Autodesk Inventor part; units mm, degrees
ref_plane "YZ Plane" through (0, 0, 0) normal (1, 0, 0) x (0, 1, 0)
ref_plane "XZ Plane" through (0, 0, 0) normal (0, 1, 0) x (-1, 0, 0)
ref_plane "XY Plane" through (0, 0, 0) normal (0, 0, 1) x (1, 0, 0)
sketch "Sketch1" plane through (0, 0, 0) normal (0, 1, 0) x (-1, 0, 0)
  line L0 (-13, -110) -> (13, -110)
  line L1 (13, -110) -> (13, 110)
  line L2 (13, 110) -> (-13, 110)
  line L3 (-13, 110) -> (-13, -110)
  line L4 (-13, -110) -> (13, 110) construction
  line L5 (13, -110) -> (-13, 110) construction
  point P0 (0, 0)
  dimension "d0" = 220
  dimension "d1" = 26
extrude "Extrusion1" add sketch "Sketch1" along normal blind 10
sketch "Sketch3" plane through (0, 0, 0) normal (0, -1, 0) x (1, 0, 0)
  line L0 (13, 110) -> (13, -110)
  line L1 (-13, -14) -> (13, -14)
  line L2 (13, -14) -> (13, 14)
  line L3 (13, 14) -> (-13, 14)
  line L4 (-13, 14) -> (-13, -14)
  line L5 (-13, -14) -> (13, 14) construction
  line L6 (13, -14) -> (-13, 14) construction
  point P0 (0, 0)
  dimension "d4" = 28
extrude "Extrusion2" add sketch "Sketch3" along normal blind 10
sketch "Sketch4" plane through (0, -10, 0) normal (0, -1, 0) x (1, 0, 0)
  line L0 (-10.125, 10.125) -> (10.125, 10.125)
  line L1 (10.125, 10.125) -> (10.125, -10.125)
  line L2 (10.125, -10.125) -> (-10.125, -10.125)
  line L3 (-10.125, -10.125) -> (-10.125, 10.125)
  line L4 (-10.125, 10.125) -> (10.125, -10.125) construction
  line L5 (10.125, 10.125) -> (-10.125, -10.125) construction
  point P0 (0, 0)
  dimension "d7" = 20.25
  dimension "d8" = 20.25
extrude "Extrusion3" cut sketch "Sketch4" against normal through all
sketch "Sketch5" plane through (-13, 0, 110) normal (-1, 0, 0) x (0, 0, 1)
  point P0 (-110, 0)
hole "Hole1" at (-13, 0, 0) direction (1, 0, 0) diameter 4.3 end through all
sketch "Sketch6" plane through (-13, 0, 110) normal (-1, 0, 0) x (0, 0, 1)
  circle A0 centre (-35, 0) radius 6.6
  line L0 (-96, 0) -> (0, 0)
  point P0 (-110, 0)
  dimension "d18" = 75
  dimension "d19" = 13.2
extrude "Extrusion4" cut sketch "Sketch6" against normal through all
sketch "Sketch7" plane through (0, 0, 0) normal (0, -1, 0) x (1, 0, 0)
  line L0 (-13, 81.6) -> (13, 81.6)
  line L1 (-13, 68.4) -> (-13, 81.6)
  line L2 (13, 68.4) -> (-13, 68.4)
  line L3 (13, 81.6) -> (13, 68.4)
  line L4 (0, 85) -> (0, 65)
  point P0 (0, 0)
  point P1 (0, 75)
  point P2 (13, 75)
  point P3 (0, 68.4)
  dimension "d22" = 20
hole "Hole2" at (0, 0, 65) at (0, 0, 85) direction (0, 1, 0) diameter 2.459 end through all
pattern_linear "Rectangular Pattern1" count 2 spacing 20 along (0, 0, 1) count 2 spacing 20 along (0, 0, -1) of "Extrusion4"
pattern_linear "Rectangular Pattern2" count 2 spacing 20 along (0, 0, 1) count 2 spacing 20 along (0, 0, -1) of "Hole2"
mirror "Mirror1" about plane through (0, 0, 0) normal (0, 0, 1) of "Extrusion4", "Hole2", "Rectangular Pattern1", "Rectangular Pattern2"
fillet "Fillet1" radius 5 2 edges at (0, 0, 14) (0, 0, -14)
properties part number "holder"
Geometry check sheet. Reference: the model listing, model coordinates, mm. A direction names the side the tool comes from. Coordinates: 2 decimals unless noted, no trailing zeros. Order: outer loops, then holes, each group sorted by start corner. A loop starts at its lowest first (then second) coordinate and runs counter-clockwise, first axis right, second up. Notation, with made-up numbers: (-4.75, 80) - (32.25, 80) arc R28 ccw to (32.25, 99) - close; hole circle Ø4 at (41, -35.75). An arc over 180 degrees is marked (long way). Answer in a Markdown table with one row per item. Add a question column.
1. Section check A-A (x = -3.5). Enter the section's corners in (y, z) (3 decimals), plus the area to 3 significant figures.
2. Material ranges on L1, parallel to X at y = 5.5, z = -85; L2, parallel to Y at x = 0.5, z = 33.5; L3, parallel to Z at x = -0.5, y = -6.75 (3 decimals), recorded low to high. Write a range as [from, to].
3. Gauge pin test, flat ends, axial feed: pin 1 Ø3 at (x, z) = (0, -105) entering from +Y; pin 2 Ø4 at (x, y) = (1, -6.5) entering from +Z; pin 3 Ø3.5 at (x, z) = (1.5, -64) entering from -Y; pin 4 Ø8 at (x, z) = (-2.5, 21.5) entering from -Y. Record the tip position at first contact, or that the pin passes through.
4. Draft check along Z on faces 1 (the face through (0, -1, -16)), 2 (the face through (0.2, 0, 83.5)), 3 (the face through (-10.125, -2.4, -0.1)). Enter one of: +Z half, -Z half, draft (parallel to the pull), parting line (faces both ways), or undercut.
5. Section check B-B (z = 75). Enter the section's corners in (x, y).
6. Access from +Z, -Z, +X, -X, +Y, -Y to the whole of each face (thin tool, end or side, straight path). Record for faces 4 (the face through (10.125, -2.4, 0.1)), 5 (the face through (-13, 5, -1)), 6 (the face through (0, -7, -14)), 7 (the face through (0, 0, 107)).
7. Section check C-C (z = -35). Enter the section's corners in (x, y), plus the area to 3 significant figures.
Data:
| question | item | result |
|---|---|---|
| 1 | outline | (-10, -14) - (-5, -14) arc R5 cw to (0, -19) - (0, -48.4) arc R6.6 cw to (0, -61.6) - (0, -68.4) arc R6.6 cw to (0, -81.6) - (0, -88.4) arc R6.6 cw to (0, -101.6) - (0, -110) - (10, -110) - (10, -10.125) - (-10, -10.125) - close; (-10, 10.125) - (10, 10.125) - (10, 110) - (0, 110) - (0, 101.6) arc R6.6 cw to (0, 88.4) - (0, 81.6) arc R6.6 cw to (0, 68.4) - (0, 61.6) arc R6.6 cw to (0, 48.4) - (0, 19) arc R5 cw to (-5, 14) - (-10, 14) - close |
| 1 | area | 1,680 mm² |
| 2 | L1 | x = [-13, -1.23], [1.23, 13] |
| 2 | L2 | y = [0, 10] |
| 2 | L3 | z = [-14, -10.125], [10.125, 14] |
| 3 | pin 1 | stops at y = 10 |
| 3 | pin 2 | stops at z = 14.03 |
| 3 | pin 3 | stops at y = 0 |
| 3 | pin 4 | stops at y = -0.23 |
| 4 | face 1 | -Z half |
| 4 | face 2 | draft |
| 4 | face 3 | undercut |
| 5 | outline | (-13, 6.6) - (13, 6.6) - (13, 10) - (-13, 10) - close |
| 6 | face 4 | +Y, -Y |
| 6 | face 5 | +Z, -Z, -X, +Y, -Y |
| 6 | face 6 | -Z, +X, -X, -Y |
| 6 | face 7 | +Z, +X, -X, -Y |
| 7 | outline | (-13, 0) - (13, 0) - (13, 10) - (-13, 10) - close |
| 7 | area | 260 mm² |
